from build123d import *

# Parameters (mm, degrees)
F0_W      = 76.2
F0_H      = 90
F1_DEPTH  = 25.4
F2_R      = 9.55
F2_R_2    = 4
F3_DEPTH  = 25.4
F5_R      = 1.5
F6_DEPTH  = 15
F7_W      = 95.184714
F7_H      = 99.811753
F7_R      = 30
F8_DEPTH  = 1.6
F9_R      = 24
F10_DEPTH = 8
F11_R     = 32.25
F12_DEPTH = 9
F13_R     = 1


with BuildPart() as f1:
    # F0 (on Top) → F1 (new body)
    with BuildSketch(Plane.XY):
        with Locations((38.1, 45)):
            Rectangle(F0_W, F0_H)
    extrude(amount=F1_DEPTH)

    # F2 (on face) → F3 (cut, through all)
    with BuildSketch(Plane.XY.offset(25.4)):
        with Locations((38.1, 54)):
            Circle(F2_R)
        with Locations((12.1, 10)):
            Circle(F2_R_2)
        with Locations((64.1, 10)):
            Circle(F2_R_2)
    extrude(amount=-F3_DEPTH, mode=Mode.SUBTRACT)

    # F5 (on face) → F6 (cut)
    with BuildSketch(Plane.XY.offset(25.4)):
        with Locations((8.1, 84)):
            Circle(F5_R)
        with Locations((68.1, 84)):
            Circle(F5_R)
        with Locations((68.1, 24)):
            Circle(F5_R)
        with Locations((8.1, 24)):
            Circle(F5_R)
    extrude(amount=-F6_DEPTH, mode=Mode.SUBTRACT)

    # F7 (on face) → F8 (cut)
    with BuildSketch(Plane.XY.offset(25.4)):
        with Locations((40.338032, 44.112226)):
            Rectangle(F7_W, F7_H)
        with Locations((38.1, 54)):
            Circle(F7_R, mode=Mode.SUBTRACT)
    extrude(amount=-F8_DEPTH, mode=Mode.SUBTRACT)

    # F9 (on face) → F10 (cut)
    with BuildSketch(Plane.XY.offset(25.4)):
        with Locations((38.1, 54)):
            Circle(F9_R)
    extrude(amount=-F10_DEPTH, mode=Mode.SUBTRACT)

    # F11 (on face) → F12 (cut)
    with BuildSketch(Plane(origin=(0, 0, 0), x_dir=(1, 0, 0), z_dir=(0, 0, -1))):
        with Locations((38.1, -54)):
            Circle(F11_R)
    extrude(amount=-F12_DEPTH, mode=Mode.SUBTRACT)

    # F13
    f13_edges = [f1.edges().sort_by_distance(p)[0] for p in [
        (76.2, 0, 11.9),
        (0, 0, 11.9),
        (76.2, 90, 11.9),
        (0, 90, 11.9),
    ]]
    fillet(f13_edges, radius=F13_R)


solid = f1.part
Verification items for the finished model (mm, model axes). A direction names the side the tool comes from. Give positions to 0.01 mm unless a question says otherwise; leave off trailing zeros. Write each loop counter-clockwise with the first axis right and the second up, starting at its lowest first coordinate (ties: lowest second). Pieces come first, ordered by that corner, then holes. Notation, with made-up numbers: M -1,75.5 L 53,75.5 A26 ccw 53,107.5 Z; hole C 1,11 d2. An arc over 180 degrees is marked long. Put each result on its own line as item: value. Start each with the question number.
1. Section check B-B (z = 22). Record the cut outline in (x, y), and give its area (3 significant figures).
2. Go/stop test with flat-tipped pins: pin 1 Ø2.5 at (x, y) = (8, 84.5) entering from +Z; pin 2 Ø11.5 at (x, y) = (38.1, 54) entering from +Z; pin 3 Ø4 at (x, y) = (23, 68) entering from -Z; pin 4 Ø1.5 at (x, y) = (67.5, 84) entering from +Z. Record where each tip stops, or that it passes through.
3. Scan lines: line 1 along X through (y, z) = (84, 18.75); line 2 along Y through (x, z) = (64.1, 9.5); line 3 along X through (y, z) = (53, 3.75). Record each from-to range of solid material in increasing order. Write a range as [from, to].
4. Section check A-A (y = 10). Record the cut outline in (x, z), and give its area (3 significant figures).
5. Set-up check for faces 1 (the face through (9.15, 12.7, 12.07)), 2 (the face through (30, 61, 9)), 3 (the face through (68, 24, 10.4)): record each of +Z, -Z, +X, -X, +Y, -Y from which the full face is reachable in a straight line by a thin tool's end or side.
6. Draft check along X on faces 4 (the face through (8.906, 25.265, 17.194)), 5 (the face through (38, 90, 12)), 6 (the face through (38, 44, 17.4)), 7 (the face through (76.2, 44, 12)). Enter one of: +X half, -X half, draft (parallel to the pull), parting line (faces both ways), or undercut.
7. Section check D-D (y = 54). Record the cut outline in (x, z).
8. Section check C-C (x = 30). Record the cut outline in (y, z).
Answer list:
1. outline: M 0,1 A1 ccw 1,0 L 75.2,0 A1 ccw 76.2,1 L 76.2,89 A1 ccw 75.2,90 L 1,90 A1 ccw 0,89 Z; hole C 8.1,24 d3; hole C 8.1,84 d3; hole C 12.1,10 d8; hole C 38.1,54 d48; hole C 64.1,10 d8; hole C 68.1,24 d3; hole C 68.1,84 d3
1. area: 4,920 mm2
2. pin 1: z = 23.8
2. pin 2: through
2. pin 3: z = 9
2. pin 4: z = 10.4
3. line 1: [0, 6.6], [9.6, 66.6], [69.6, 76.2]
3. line 2: [0, 6], [14, 90]
3. line 3: [0, 5.87], [70.33, 76.2]
4. outline: M 0,0 L 8.1,0 L 8.1,23.8 L 0,23.8 Z; M 16.1,0 L 60.1,0 L 60.1,23.8 L 16.1,23.8 Z; M 68.1,0 L 76.2,0 L 76.2,23.8 L 68.1,23.8 Z
4. area: 1,430 mm2
5. face 1: +Z, -Z
5. face 2: -Z
5. face 3: +Z
6. face 4: undercut
6. face 5: draft
6. face 6: undercut
6. face 7: +X half
7. outline: M 0,0 L 5.85,0 L 5.85,9 L 28.55,9 L 28.55,17.4 L 14.1,17.4 L 14.1,25.4 L 8.1,25.4 L 8.1,23.8 L 0,23.8 Z; M 47.65,9 L 70.35,9 L 70.35,0 L 76.2,0 L 76.2,23.8 L 68.1,23.8 L 68.1,25.4 L 62.1,25.4 L 62.1,17.4 L 47.65,17.4 Z
8. outline: M 0,0 L 22.78,0 L 22.78,9 L 48.94,9 L 48.94,17.4 L 31.41,17.4 L 31.41,25.4 L 25.11,25.4 L 25.11,23.8 L 0,23.8 Z; M 59.06,9 L 85.22,9 L 85.22,0 L 90,0 L 90,23.8 L 82.89,23.8 L 82.89,25.4 L 76.59,25.4 L 76.59,17.4 L 59.06,17.4 Z
